Read the model definition and answer for the solid it produces. Units are mm, in the model's axes. Face numbers are marked on the shaded views. A direction names the side the tool comes from. Give positions to 0.01 mm unless a question says otherwise; leave off trailing zeros. Loops run counter-clockwise (first coordinate to the right, second up) from the corner with the lowest first, then second, coordinate; pieces in that order, holes last. Notation, with made-up numbers: M 29,48.5 L 59,48.5 A19 ccw 59,52.5 Z; hole C 61.5,51 d8. An arc over 180 degrees is marked long. Return JSON: item names as keys, results as strings. Group by question number.
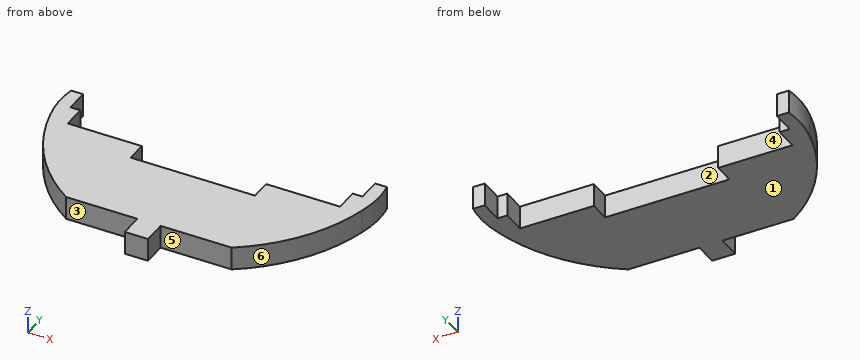
```python
from build123d import *

# Parameters (mm, degrees)
BOSS_EXTRUDE1_DEPTH = 3


with BuildPart() as part:
    # Sketch1 → Boss-Extrude1 (new body)
    with BuildSketch(Plane.XY):
        with BuildLine():
            Line((8.024, 16.106), (8.024, 13.464))
            Line((8.024, 13.464), (-8.024, 13.464))
            Line((-8.024, 13.464), (-8.024, 16.106))
            Line((-8.024, 16.106), (-17.583, 16.106))
            Line((-17.583, 16.106), (-17.583, 19.106))
            Line((-17.583, 19.106), (-18.859, 19.106))
            Line((-18.859, 19.106), (-18.859, 22.106))
            Line((-18.859, 22.106), (-20.394542528, 22.106))
            ThreePointArc((-20.394542528, 22.106), (-20.571042392, 19.357451914), (-20.154, 16.635))
            ThreePointArc((-20.154, 16.635), (-16.727003231, 8.90904451), (-10.684, 3))
            Line((-10.684, 3), (-1.5, 3))
            Line((-1.5, 3), (-1.5, 0))
            Line((-1.5, 0), (1.5, 0))
            Line((1.5, 0), (1.5, 3))
            Line((1.5, 3), (10.684, 3))
            ThreePointArc((10.684, 3), (16.727003231, 8.90904451), (20.154, 16.635))
            ThreePointArc((20.154, 16.635), (20.571042392, 19.357451914), (20.394542528, 22.106))
            Line((20.394542528, 22.106), (18.859, 22.106))
            Line((18.859, 22.106), (18.859, 19.106))
            Line((18.859, 19.106), (17.583, 19.106))
            Line((17.583, 19.106), (17.583, 16.106))
            Line((17.583, 16.106), (8.024, 16.106))
        make_face()
    extrude(amount=BOSS_EXTRUDE1_DEPTH)


solid = part.part
```
1. Find section A-A (z = 1.3). Write down the section's boundary in (x, y) (3 decimals).
2. Find section B-B (y = 18.5). Write down the section's boundary in (x, z), and give its area (3 significant figures).
3. Find section D-D (y = 8.25). Write down the section's boundary in (x, z).
4. Flat-ended cylindrical pins translate along their axes: P1, Ø1.3, axis at y = 15, z = 2, coming from the +X side; P2, Ø0.9, axis at x = -12.5, z = 1.5, coming from the +Y side; P3, Ø1, axis at y = 15, z = 1, coming from the -X side. Find the tip coordinate at first contact, or state that the pin passes through.
5. Straight lines are drawn through the part: line 1 along X through (y, z) = (19.5, 0.3); line 2 along X through (y, z) = (17.75, 1.3); line 3 along Y through (x, z) = (9, 1.05). For each, find the intervals that lie inside material, in ascending order.
6. For the marked faces 1, 2 and 3, determine the directions among +Z, -Z, +X, -X, +Y, -Y from which every point of the face is accessible in a straight line to the end or side of a thin tool.
7. The mould has two halves that part along X. Classify the marked faces 4, 5 and 6: +X half, -X half, draft (parallel to the pull), parting line (faces both ways), or undercut.
8. Find section C-C (x = -0.5). Write down the section's boundary in (y, z).
Result:
{
 "1": {"outline": "M -20.395,22.106 A12.768 ccw -20.154,16.635 A22.428 ccw -10.684,3 L -1.5,3 L -1.5,0 L 1.5,0 L 1.5,3 L 10.684,3 A22.428 ccw 20.154,16.635 A12.768 ccw 20.395,22.106 L 18.859,22.106 L 18.859,19.106 L 17.583,19.106 L 17.583,16.106 L 8.024,16.106 L 8.024,13.464 L -8.024,13.464 L -8.024,16.106 L -17.583,16.106 L -17.583,19.106 L -18.859,19.106 L -18.859,22.106 Z"},
 "2": {"outline": "M -20.5,0 L -17.58,0 L -17.58,3 L -20.5,3 Z; M 17.58,0 L 20.5,0 L 20.5,3 L 17.58,3 Z", "area": "17.5 mm2"},
 "3": {"outline": "M -16.25,0 L 16.25,0 L 16.25,3 L -16.25,3 Z"},
 "4": {"P1": "stops at x = 19.9", "P2": "stops at y = 16.11", "P3": "stops at x = -19.86"},
 "5": {"line 1": "x = -20.58 to -18.86, 18.86 to 20.58", "line 2": "x = -20.4 to -17.58, 17.58 to 20.4", "line 3": "y = 3 to 16.11"},
 "6": {"face 1": "-Z, +X, -X, +Y, -Y", "face 2": "+Z, -Z, +Y", "face 3": "+Z, -Z, -X, -Y"},
 "7": {"face 4": "undercut", "face 5": "draft", "face 6": "+X half"},
 "8": {"outline": "M 0,0 L 13.46,0 L 13.46,3 L 0,3 Z"}
}
